Geometry: final body of the model. Coordinates: model frame, mm. A direction names the side the tool comes from. Give positions to 0.01 mm unless a question says otherwise; leave off trailing zeros. Loops run counter-clockwise (first coordinate to the right, second up) from the corner with the lowest first, then second, coordinate; pieces in that order, holes last. Notation, with made-up numbers: (27.5, 58.5) -> (51.5, 58.5) arc R9 ccw to (51.5, 66.5) -> close; hole circle Ø8 at (4, 7). An arc over 180 degrees is marked (long way). Answer in a Markdown table with one row per item. Add a question column.
1) Access query for faces 1 (the flat face through (14.75, 0, -5)), 2 (the flat face through (-14.75, 0, 2)), 3 (the flat face through (0, -5, -9)). Directions: +Z, -Z, +X, -X, +Y, -Y. A direction counts if a zero-diameter tool reaches every point of the face in a straight line with its end or side. Return the directions, or none.
2) Section query B-B (x = 13.5). Return the cut outline in (y, z).
3) First-contact query: P1, Ø6.5, axis at x = 3, y = -4.5, coming from the +Z side; P2, Ø2, axis at x = 12.5, z = -6, coming from the +Y side; P3, Ø8, axis at x = 12, z = -7.5, coming from the -Y side. Flat tips, straight axial feed; report the tip coordinate or a pass-through.
4) Section query D-D (z = -3.5). Return the cut outline in (x, y).
5) Draft query along Y for faces 4 (the flat face through (-0.2, -16, -0.5)), 5 (the flat face through (3.295, 3.027, 3.093)), 6 (the flat face through (-0.1, 14.3, -1)). Return one class per face: +Y half, -Y half, draft (parallel to the pull), parting line (faces both ways), or undercut.
6) Line query: line 1 (X direction, y = 6, z = 3.25); line 2 (X direction, y = 2, z = 2.75); line 3 (Z direction, x = 15.5, y = -13). Output: solid intervals per line, ascending. Write a range as from..to.
7) Section query A-A (y = -4.5). Return the cut outline in (x, z) (3 decimals).
8) Section query C-C (y = -9.5). Return the cut outline in (x, z), plus the area to 3 significant figures.
Solid Edge part; units mm, degrees
sketch "Sketch1" plane through (0, 0, 0) normal (0, 0, 1) x (1, 0, 0)
  line L0 (-14.75, -14) -> (14.75, -14)
  line L1 (14.75, -14) -> (14.75, 14)
  line L2 (14.75, 14) -> (-14.75, 14)
  line L3 (-14.75, 14) -> (-14.75, -14)
extrude "Protrusion1" add sketch "Sketch1" along normal blind 4.6
sketch "Sketch2" plane through (0, 0, 0) normal (0, 0, -1) x (1, 0, 0)
  line L0 (16.75, 16) -> (16.75, -16)
  line L1 (16.75, -16) -> (-16.75, -16)
  line L2 (-16.75, -16) -> (-16.75, 16)
  line L3 (-16.75, 16) -> (16.75, 16)
extrude "ExtrudedProtrusion_2" add sketch "Sketch2" along normal blind 1
sketch "Sketch3" plane through (0, 0, 0) normal (0, 0, 1) x (1, 0, 0)
  line L0 (14.75, 14) -> (-14.75, 14)
  line L1 (-14.75, 14) -> (-14.75, -14)
  line L2 (-14.75, -14) -> (14.75, -14)
  line L3 (14.75, -14) -> (14.75, 14)
extrude "ExtrudedProtrusion_3" add sketch "Sketch3" against normal blind 9.5
sketch "Sketch4" plane through (0, 0, 4.6) normal (0, 0, 1) x (1, 0, 0)
  line L0 (-13.25, 12.5) -> (-13.25, -12.5)
  line L1 (-13.25, -12.5) -> (13.25, -12.5)
  line L2 (13.25, -12.5) -> (13.25, 12.5)
  line L3 (13.25, 12.5) -> (-13.25, 12.5)
extrude "ExtrudedCutout_1" cut sketch "Sketch4" against normal blind 2
chamfer "Chamfer_1" distance 2.5 angle 45 4 edges at (0, 12.5, 2.6) (13.25, 0, 2.6) (0, -12.5, 2.6) (-13.25, 0, 2.6)
sketch "Sketch5" plane through (0, 0, 2.6) normal (0, 0, 1) x (1, 0, 0)
  line L0 (-6.5, -8.9305) -> (6.5, -8.9305)
  line L1 (6.5, -8.9305) -> (6.5, 0.0695)
  line L2 (6.5, 0.0695) -> (0, 6.0695)
  line L3 (0, 6.0695) -> (-6.5, 0.0695)
  line L4 (-6.5, 0.0695) -> (-6.5, -8.9305)
  line L5 (8.4502, 1.1302) -> (0, 8.9305)
  line L6 (0, 8.9305) -> (-8.4502, 1.1302)
  line L7 (-8.4502, 1.1302) -> (-8.4502, -0.3698)
  line L8 (-8.4502, -0.3698) -> (0, 7.4305)
  line L9 (0, 7.4305) -> (8.4502, -0.3698)
  line L10 (8.4502, -0.3698) -> (8.4502, 1.1302)
extrude "ExtrudedProtrusion_4" add sketch "Sketch5" along normal blind 1
sketch "Sketch6" plane through (0, 0, -9.5) normal (0, 0, -1) x (-1, 0, 0)
  line L0 (7.375, -5) -> (7.375, 5)
  line L1 (7.375, 5) -> (-7.375, 5)
  line L2 (-7.375, 5) -> (-7.375, -5)
  line L3 (-7.375, -5) -> (7.375, -5)
extrude "ExtrudedCutout_2" cut sketch "Sketch6" against normal blind 1
properties material "Polycarbonate"
Evaluation:
| question | item | result |
|---|---|---|
| 1 | face 1 | -Z, +X, +Y, -Y |
| 1 | face 2 | +Z, -X, +Y, -Y |
| 1 | face 3 | -Z |
| 2 | outline | (-16, -1) -> (-14, -1) -> (-14, -9.5) -> (14, -9.5) -> (14, -1) -> (16, -1) -> (16, 0) -> (14, 0) -> (14, 4.6) -> (-14, 4.6) -> (-14, 0) -> (-16, 0) -> close |
| 3 | P1 | z = 3.6 |
| 3 | P2 | y = 14 |
| 3 | P3 | y = -14 |
| 4 | outline | (-14.75, -14) -> (14.75, -14) -> (14.75, 14) -> (-14.75, 14) -> close |
| 5 | face 4 | -Y half |
| 5 | face 5 | undercut |
| 5 | face 6 | draft |
| 6 | line 1 | -14.75..-11.4, -3.17..-1.55, -0.08..0.08, 1.55..3.17, 11.4..14.75 |
| 6 | line 2 | -14.75..-10.9, -7.51..-5.88, -4.41..4.41, 5.88..7.51, 10.9..14.75 |
| 6 | line 3 | -1..0 |
| 7 | outline | (-16.75, -1) -> (-14.75, -1) -> (-14.75, -9.5) -> (-7.375, -9.5) -> (-7.375, -8.5) -> (7.375, -8.5) -> (7.375, -9.5) -> (14.75, -9.5) -> (14.75, -1) -> (16.75, -1) -> (16.75, 0) -> (14.75, 0) -> (14.75, 4.6) -> (12.75, 4.6) -> (10.75, 2.6) -> (6.5, 2.6) -> (6.5, 3.6) -> (-6.5, 3.6) -> (-6.5, 2.6) -> (-10.75, 2.6) -> (-12.75, 4.6) -> (-14.75, 4.6) -> (-14.75, 0) -> (-16.75, 0) -> close |
| 8 | outline | (-16.75, -1) -> (-14.75, -1) -> (-14.75, -9.5) -> (14.75, -9.5) -> (14.75, -1) -> (16.75, -1) -> (16.75, 0) -> (14.75, 0) -> (14.75, 4.6) -> (12.75, 4.6) -> (10.75, 2.6) -> (-10.75, 2.6) -> (-12.75, 4.6) -> (-14.75, 4.6) -> (-14.75, 0) -> (-16.75, 0) -> close |
| 8 | area | 373 mm² |
